Verification items for this drawing (mm, ordinates from the low corner). Coordinates: 2 decimals unless noted, no trailing zeros. Write each loop counter-clockwise with the first axis right and the second up, starting at its lowest first coordinate (ties: lowest second). Pieces come first, ordered by that corner, then holes. Notation, with made-up numbers: M 73,-15.75 L 108,-15.75 A25 ccw 108,21.25 Z; hole C 6.5,-20.5 d7. An arc over 180 degrees is marked long. Write each question's results on one line, items separated by ' | '.
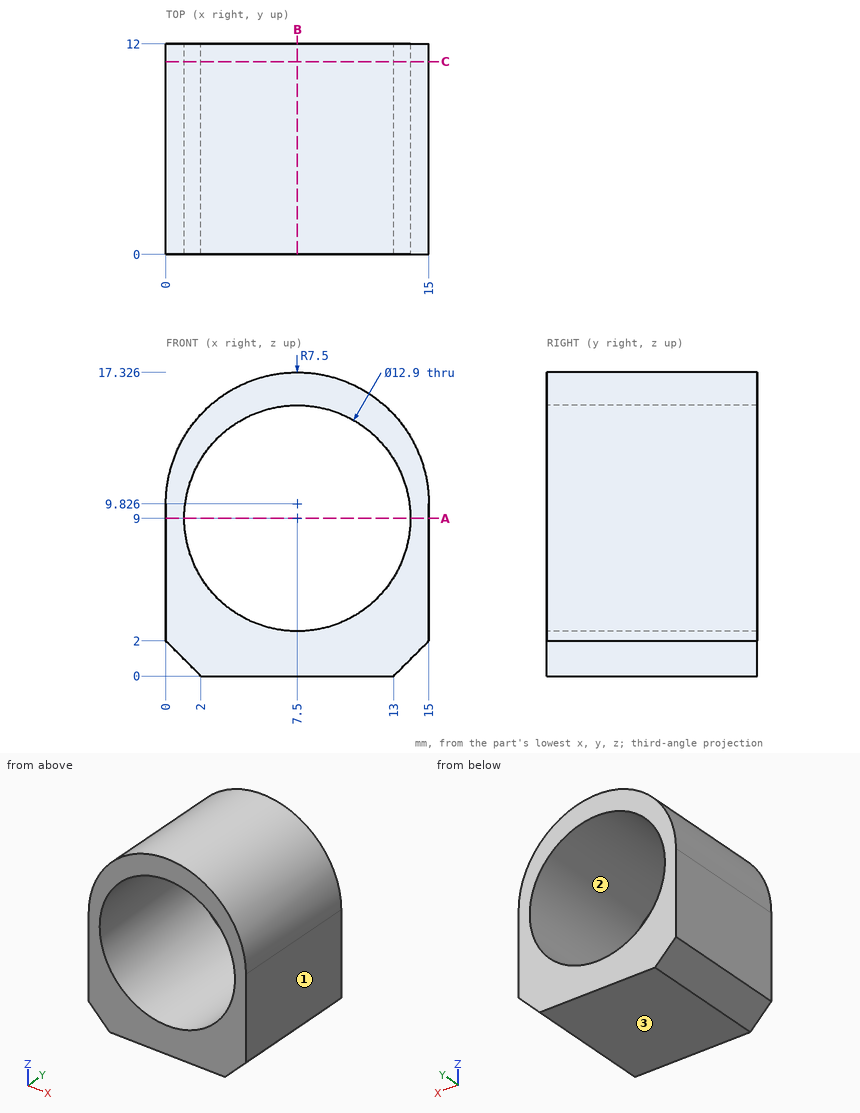
Q1. Sectioned sample at B-B on x = 7.5. Record the cut outline in (y, z).
Geometry check:
outline: M 0,0 L 12,0 L 12,2.55 L 0,2.55 Z; M 0,15.45 L 12,15.45 L 12,17.33 L 0,17.33 Z
Q2. Sectioned sample at A-A on z = 9. Record the cut outline in (x, y), and give its area (3 significant figures).
Geometry check:
outline: M 0,0 L 1.05,0 L 1.05,12 L 0,12 Z; M 13.95,0 L 15,0 L 15,12 L 13.95,12 Z | area: 25.2 mm2
Q3. Scan lines: probe 1 along Z at (x, y) = (7.5, 5); probe 2 along X at (y, z) = (2, 8.75) (1 decimal); probe 3 along X at (y, z) = (4.25, 3.25) (1 decimal). Record each from-to range of solid material in increasing order.
Geometry check:
probe 1: z = 0 to 2.55, 15.45 to 17.33 | probe 2: x = 0 to 1.1, 13.9 to 15 | probe 3: x = 0 to 4.6, 10.4 to 15
Q4. Mould release check, pull along Z, two halves, no side actions. Record for the marked faces 1, 2 and 3: pulls with the +Z half, pulls with the -Z half, needs draft (parallel to the pull), parting line crosses it, or undercut.
Geometry check:
face 1: needs draft | face 2: undercut | face 3: pulls with the -Z half
Q5. Depth check by flat-ended pin: P1, Ø7.5, axis at x = 7.5, z = 9, coming from the +Y side; P2, Ø1.5, axis at x = 4.5, y = 5, coming from the +Z side; P3, Ø4, axis at y = 3.5, z = 14.5, coming from the -X side; P4, Ø2, axis at x = 9, y = 7, coming from the +Z side. Enter the tip coordinate at first touch or a pass-through.
Geometry check:
P1: passes through | P2: stops at z = 16.98 | P3: stops at x = 0.49 | P4: stops at z = 17.31
Q6. Sectioned sample at C-C on y = 11. Record the cut outline in (x, z), and give its area (3 significant figures).
Geometry check:
outline: M 0,2 L 2,0 L 13,0 L 15,2 L 15,9.83 A7.5 ccw 0,9.83 Z; hole C 7.5,9 d12.9 | area: 101 mm2
